Print and shaded views of the part. All mm, measured from the part's lowest x, y and z. Round coordinates to 2 decimals unless told otherwise and drop trailing zeros. Loops run counter-clockwise (first coordinate to the right, second up) from the corner with the lowest first, then second, coordinate; pieces in that order, holes last. Notation, with made-up numbers: (-9, 4) -> (42, 4) arc R8 ccw to (42, 15) -> close; hole circle Ø10 at (-15, -24). An arc over 180 degrees is marked (long way). Use a Markdown table: item, result.
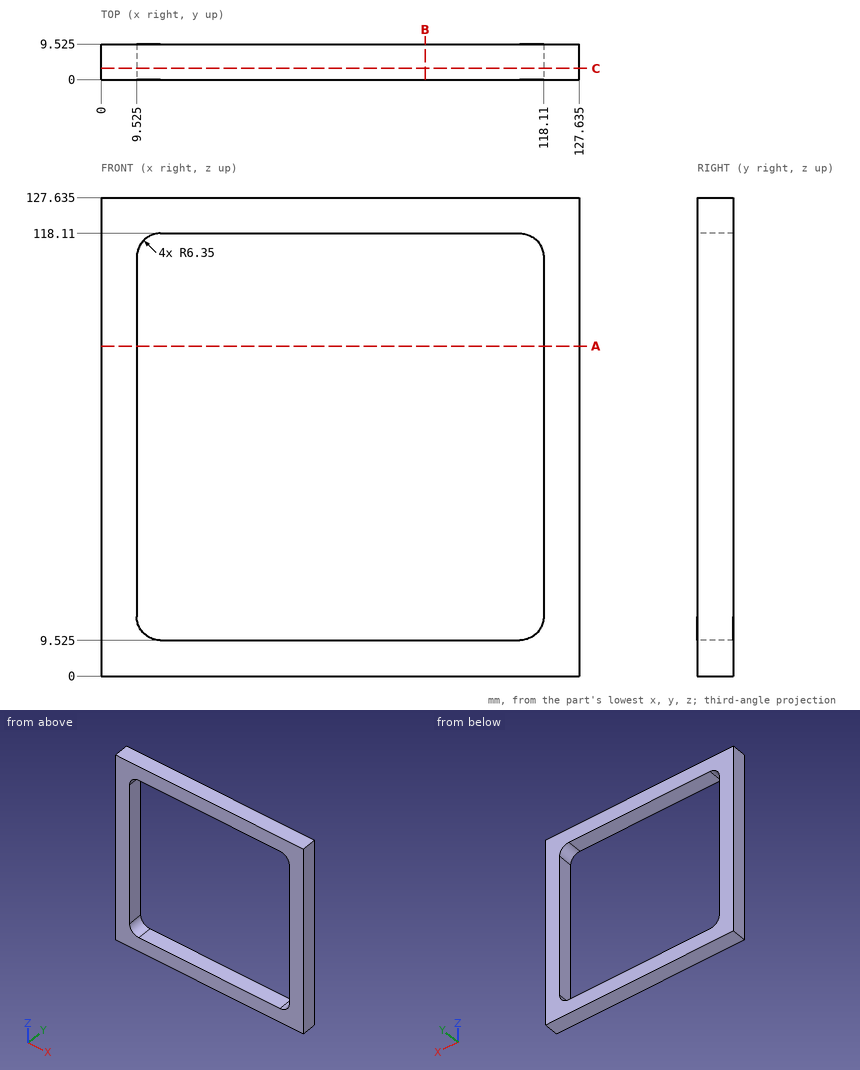
Q1. Drill centre lines: L1, parallel to Z at x = 43.5, y = 9 (3 decimals); L2, parallel to X at y = 8.75, z = 112.5 (3 decimals). Where is each one in solid material? Low to high. Write a range as from..to.
Results list:
| item | result |
|---|---|
| L1 | z = 0..9.525, 118.11..127.635 |
| L2 | x = 0..9.568, 118.067..127.635 |
Q2. Band-saw the part on C-C, the plane y = 3. Give the cut face in (x, z) (3 decimals), plus the area to 3 significant figures.
Results list:
| item | result |
|---|---|
| outline | (0, 0) -> (127.635, 0) -> (127.635, 127.635) -> (0, 127.635) -> close; hole (9.525, 15.875) arc R6.35 ccw to (15.875, 9.525) -> (111.76, 9.525) arc R6.35 ccw to (118.11, 15.875) -> (118.11, 111.76) arc R6.35 ccw to (111.76, 118.11) -> (15.875, 118.11) arc R6.35 ccw to (9.525, 111.76) -> close |
| area | 4,530 mm² |
Q3. Band-saw the part on A-A, the plane z = 88. Give the cut face in (x, y) (3 decimals).
Results list:
| item | result |
|---|---|
| outline | (0, 0) -> (9.525, 0) -> (9.525, 9.525) -> (0, 9.525) -> close; (118.11, 0) -> (127.635, 0) -> (127.635, 9.525) -> (118.11, 9.525) -> close |
Q4. Band-saw the part on B-B, the plane x = 86.5. Give the cut face in (y, z) (3 decimals).
Results list:
| item | result |
|---|---|
| outline | (0, 0) -> (9.525, 0) -> (9.525, 9.525) -> (0, 9.525) -> close; (0, 118.11) -> (9.525, 118.11) -> (9.525, 127.635) -> (0, 127.635) -> close |
